Could you check a few things on this model? Use its own coordinates, in mm. Face numbers are marked on the shaded views. A direction names the side the tool comes from. Give positions to 0.01 mm unless a question says otherwise; leave off trailing zeros. Order: outer loops, then holes, each group sorted by start corner. A loop starts at its lowest first (then second) coordinate and runs counter-clockwise, first axis right, second up. Notation, with made-up numbers: (-21, 89) -> (31, 89) arc R19 ccw to (31, 100) -> close; hole circle Ø8 at (64, 42.5). An arc over 180 degrees is marked (long way). Write each question's results on one line, items separated by ' | '.
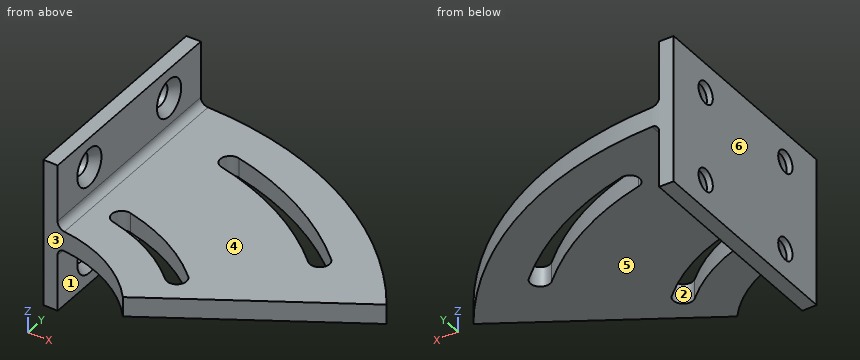
```python
from build123d import *

# Parameters (mm, degrees)
BOSS_EXTRUDE1_DEPTH                               = 2
BOSS_EXTRUDE2_DEPTH                               = 15
CSK_FOR_8_FLAT_HEAD_SOCKET_CAP_SCREW1_D           = 4.4958
CSK_FOR_8_FLAT_HEAD_SOCKET_CAP_SCREW1_DEPTH       = 15
CSK_FOR_8_FLAT_HEAD_SOCKET_CAP_SCREW1_CSINK_D     = 7.62
CSK_FOR_8_FLAT_HEAD_SOCKET_CAP_SCREW1_CSINK_ANGLE = 82
CSK_FOR_8_FLAT_HEAD_SOCKET_CAP_SCREW1_TIP         = 0.7087601475210669
FILLET1_R                                         = 1.5


with BuildPart() as part:
    # Sketch1 → Boss-Extrude1 (new, symmetric)
    with BuildSketch(Plane.XY):
        with BuildLine():
            ThreePointArc((3.0000000000000036, 29.84962311319859), (14.561896892531825, 26.228823055777227), (23.748786379167363, 18.330170362456368))
            Line((23.748786379167367, 18.33017036245637), (62.85946345754006, 40.910730301843614))
            ThreePointArc((62.859463457540045, 40.910730301843614), (37.065679841305055, 65.20073142152523), (2.9999999999999964, 74.93997598078077))
            Line((2.999999999999999, 74.93997598078074), (3, 29.849623113198593))
        make_face()
        with BuildLine():
            ThreePointArc((10.870399894306182, 40.568884704140785), (21.000000000000167, 36.373066958946325), (29.698484809835048, 29.698484809834948))
            ThreePointArc((29.698484809835044, 29.698484809834945), (29.69848480983504, 26.870057685088753), (26.87005768508885, 26.870057685088756))
            ThreePointArc((26.870057685088845, 26.87005768508876), (19.000000000000156, 32.90896534380858), (9.835123713896072, 36.70518139898452))
            ThreePointArc((9.835123713896072, 36.70518139898452), (8.420910151522994, 39.15467114176771), (10.870399894306184, 40.568884704140785))
        make_face(mode=Mode.SUBTRACT)
        with BuildLine():
            ThreePointArc((17.340876021869384, 64.71703036136746), (33.500000000000284, 58.023702053557244), (47.37615433949878, 47.37615433949861))
            ThreePointArc((47.37615433949877, 47.3761543394986), (47.376154339498754, 44.547727214752406), (44.54772721475256, 44.54772721475241))
            ThreePointArc((44.54772721475258, 44.54772721475243), (31.50000000000025, 54.55960043841949), (16.30559984145927, 60.85332705621119))
            ThreePointArc((16.30559984145927, 60.85332705621118), (14.891386279086177, 63.302816798994385), (17.340876021869388, 64.71703036136746))
        make_face(mode=Mode.SUBTRACT)
    extrude(amount=BOSS_EXTRUDE1_DEPTH, both=True)

    # Sketch1<3> → Boss-Extrude2 (add, symmetric)
    with BuildSketch(Plane.XY):
        with BuildLine():
            ThreePointArc((1.78e-15, 30), (1.501883251794565, 29.962382193309978), (3.0000000000000036, 29.84962311319859))
            Line((3, 29.849623113198593), (2.999999999999999, 74.93997598078074))
            ThreePointArc((2.9999999999999964, 74.93997598078077), (1.5003002101982155, 74.98499249369355), (-1.066e-14, 75))
            Line((0, 75), (0, 30))
        make_face()
    extrude(amount=BOSS_EXTRUDE2_DEPTH, both=True)

    # CSK for #8 Flat Head Socket Cap Screw1
    with Locations(Plane(origin=(3.0000000000000004, 6e-17, 0), x_dir=(0, 0, -1), z_dir=(1, 2e-17, 0))):
        with Locations((-9, 64.939975981), (9, 64.939975981), (9, 39.849623113), (-9, 39.849623113)):
            CounterSinkHole(CSK_FOR_8_FLAT_HEAD_SOCKET_CAP_SCREW1_D / 2, CSK_FOR_8_FLAT_HEAD_SOCKET_CAP_SCREW1_CSINK_D / 2, depth=CSK_FOR_8_FLAT_HEAD_SOCKET_CAP_SCREW1_DEPTH, counter_sink_angle=CSK_FOR_8_FLAT_HEAD_SOCKET_CAP_SCREW1_CSINK_ANGLE)
            with Locations((0, 0, -(CSK_FOR_8_FLAT_HEAD_SOCKET_CAP_SCREW1_DEPTH + CSK_FOR_8_FLAT_HEAD_SOCKET_CAP_SCREW1_TIP / 2))):  # 145° drill point
                Cone(0, CSK_FOR_8_FLAT_HEAD_SOCKET_CAP_SCREW1_D / 2, CSK_FOR_8_FLAT_HEAD_SOCKET_CAP_SCREW1_TIP, mode=Mode.SUBTRACT)

    # Fillet1
    fillet1_edges = [part.edges().sort_by_distance(p)[0] for p in [
        (2.9999999999999996, 52.39479954698967, -2),
        (2.9999999999999996, 52.39479954698967, 2),
    ]]
    fillet(fillet1_edges, radius=FILLET1_R)


solid = part.part
```
Q1. Suppose I cut it at C-C on z = -1. Please give me the cut outline in (x, y), and give its area (3 significant figures).
Here are the results:
outline: (0, 30) arc R30 cw to (23.75, 18.33) -> (62.86, 40.91) arc R75 ccw to (0, 75) -> close; hole (9.84, 36.71) arc R38 cw to (26.87, 26.87) arc R2 ccw to (29.7, 29.7) arc R42 ccw to (10.87, 40.57) arc R2 ccw to start; hole (16.31, 60.85) arc R63 cw to (44.55, 44.55) arc R2 ccw to (47.38, 47.38) arc R67 ccw to (17.34, 64.72) arc R2 ccw to start | area: 2,050 mm²
Q2. Thinking about a two-plate mould opening in X: for the marked faces 1, 2 and 3, which applies, +X half, -X half, draft (parallel to the pull), parting line (faces both ways), or undercut?
Here are the results:
face 1: +X half | face 2: undercut | face 3: -X half
Q3. I need wall thicknesses on line 1 along X through (y, z) = (52, -11); line 2 along Z through (x, y) = (16, 27); line 3 along X through (y, z) = (55, -1.5). Which ranges of each line are inside material? Lowest first, please.
Here are the results:
line 1: x = 0 to 3 | line 2: z = -2 to 2 | line 3: x = 0 to 30.72, 38.26 to 50.99
Q4. Suppose I cut it at B-B on x = 42.5. Please give me the cut outline in (y, z), and give its area (3 significant figures).
Here are the results:
outline: (29.16, -2) -> (46.51, -2) -> (46.51, 2) -> (29.16, 2) -> close; (51.8, -2) -> (61.8, -2) -> (61.8, 2) -> (51.8, 2) -> close | area: 109 mm²
Q5. Suppose I cut it at D-D on x = 54. Please give me the cut outline in (y, z).
Here are the results:
outline: (35.8, -2) -> (52.05, -2) -> (52.05, 2) -> (35.8, 2) -> close
Q6. Suppose I cut it at A-A on z = 9. Please give me the cut outline in (x, y).
Here are the results:
outline: (0, 30) arc R30 cw to (3, 29.85) -> (3, 36.04) -> (1.2, 37.6) -> (0, 37.6) -> close; (0, 42.1) -> (1.2, 42.1) -> (3, 43.66) -> (3, 61.13) -> (1.2, 62.69) -> (0, 62.69) -> close; (0, 67.19) -> (1.2, 67.19) -> (3, 68.75) -> (3, 74.94) arc R75 ccw to (0, 75) -> close
Q7. For the marked faces 4, 5 and 6, which set-ups out of +Z, -Z, +X, -X, +Y, -Y let a thin tool reach every point of the face, with its end or its side?
Here are the results:
face 4: +Z, +X, +Y, -Y | face 5: -Z, +X, +Y, -Y | face 6: +Z, -Z, -X, +Y, -Y
Q8. I'm going to push flat-ended pins straight in: pin 1 Ø2 at (y, z) = (52.5, 6) entering from +X; pin 2 Ø3 at (y, z) = (46, 0) entering from +X; pin 3 Ø6 at (y, z) = (39.85, -9) entering from +X. Where does each tip first touch, or does it pass through?
Here are the results:
pin 1: stops at x = 3 | pin 2: stops at x = 60.37 | pin 3: stops at x = 2.07
